Model file for the job. Use its own axes, mm. A direction names the side the tool comes from. Round coordinates to 2 decimals unless told otherwise and drop trailing zeros. Write each loop counter-clockwise with the first axis right and the second up, starting at its lowest first coordinate (ties: lowest second). Pieces come first, ordered by that corner, then holes. Notation, with made-up numbers: (24, 29.25) - (63, 29.25) arc R6 ccw to (63, 36.25) - close; hole circle Ø2 at (68.25, -39.75). An arc over 180 degrees is marked (long way). One line per item, written item: value.
from build123d import *

# Parameters (mm, degrees)
SKETCH1_W                       = 30
SKETCH1_H                       = 22
BOSS_EXTRUDE1_DEPTH             = 7
BOSS_EXTRUDE2_DEPTH             = 7
BOSS_EXTRUDE3_START             = 2
BOSS_EXTRUDE3_DEPTH             = 2
TAP_DRILL_FOR_M6X1_0_TAP2_D     = 5
TAP_DRILL_FOR_M6X1_0_TAP2_DEPTH = 8
TAP_DRILL_FOR_M6X1_0_TAP2_TIP   = 1.502151548


with BuildPart() as part:
    # Sketch1 → Boss-Extrude1 (new body)
    with BuildSketch(Plane(origin=(0, 0, 0), x_dir=(1, 0, 0), z_dir=(0, 1, 0))):
        with Locations((0, 3.5)):
            Rectangle(SKETCH1_W, SKETCH1_H)
        with BuildLine():
            ThreePointArc((-7.5, -2.5), (-10, -5), (-12.5, -2.5))
            Line((-12.5, -2.5), (-12.5, 2.5))
            ThreePointArc((-12.5, 2.5), (-10, 5), (-7.5, 2.5))
            Line((-7.5, 2.5), (-7.5, -2.5))
        make_face(mode=Mode.SUBTRACT)
        with BuildLine():
            ThreePointArc((12.5, -2.5), (10, -5), (7.5, -2.5))
            Line((7.5, -2.5), (7.5, 2.5))
            ThreePointArc((7.5, 2.5), (10, 5), (12.5, 2.5))
            Line((12.5, 2.5), (12.5, -2.5))
        make_face(mode=Mode.SUBTRACT)
    extrude(amount=BOSS_EXTRUDE1_DEPTH)

    # Sketch2 → Boss-Extrude2 (add)
    with BuildSketch(Plane(origin=(0, 0, -14.5), x_dir=(-1, 0, 0), z_dir=(0, 0, -1))):
        with BuildLine():
            Line((-15, 7), (15, 7))
            Line((15, 7), (43.5, 64))
            Line((43.5, 64), (43.5, 85))
            Line((43.5, 85), (27.855550733, 74.218014694))
            ThreePointArc((27.855550733, 74.218014694), (11.88121166, 46.405371431), (-19.795903133, 41.377147841))
            Line((-19.795903133, 41.377147841), (-30.5, 34))
            Line((-30.5, 34), (-15, 7))
        make_face()
    extrude(amount=-BOSS_EXTRUDE2_DEPTH)

    # Sketch3 → Boss-Extrude3 (add)
    with BuildSketch(Plane(origin=(0, 0, -14.5), x_dir=(-1, 0, 0), z_dir=(0, 0, -1)).offset(BOSS_EXTRUDE3_START)):
        with BuildLine():
            Line((-19.795903133, 41.377147841), (-30.5, 34))
            Line((-30.5, 34), (-25.504418015, 25.298018478))
            Line((-25.504418015, 25.298018478), (-3.837244639, 40.230800129))
            ThreePointArc((-3.837244639, 40.230800129), (-11.878974739, 39.935272554), (-19.795903133, 41.377147841))
        make_face()
        with BuildLine():
            Line((43.5, 85), (27.855550733, 74.218014694))
            ThreePointArc((27.855550733, 74.218014694), (26.38496828, 66.306368419), (23.246350456, 58.896521073))
            Line((23.246350456, 58.896521073), (43.5, 72.85511738))
            Line((43.5, 72.85511738), (43.5, 85))
        make_face()
    extrude(amount=-BOSS_EXTRUDE3_DEPTH)

    # Tap Drill for M6x1.0 Tap2
    with Locations(Plane(origin=(25.708369444, 37.302339978, 0), x_dir=(0.8233920666857286, -0.5674729108239484, 0), z_dir=(0.5674729108239484, 0.8233920666857286, 0))):
        with Locations((-75.680620934, 12), (-0.680620934, 12)):
            Hole(TAP_DRILL_FOR_M6X1_0_TAP2_D / 2, depth=TAP_DRILL_FOR_M6X1_0_TAP2_DEPTH)
            with Locations((0, 0, -(TAP_DRILL_FOR_M6X1_0_TAP2_DEPTH + TAP_DRILL_FOR_M6X1_0_TAP2_TIP / 2))):  # 118° drill point
                Cone(0, TAP_DRILL_FOR_M6X1_0_TAP2_D / 2, TAP_DRILL_FOR_M6X1_0_TAP2_TIP, mode=Mode.SUBTRACT)


solid = part.part
1. Mould opens along Z. For faces 1 (the face through (15, 3, -3)), 2 (the face through (0, 3, 7.5)), 3 (the face through (10, 3, 5)) say: released by +Z, released by -Z, zero draft, split by the parting line, or undercut.
Report:
face 1: zero draft
face 2: released by +Z
face 3: undercut
2. Band-saw the part on D-D on x = -10. Write the cut outline in (y, z).
Report:
outline: (0, -14.5) - (45.19, -14.5) - (45.19, -7.5) - (7, -7.5) - (7, -5) - (0, -5) - close; (0, 5) - (7, 5) - (7, 7.5) - (0, 7.5) - close
3. Tool access for faces 4 (the face through (-10, 3, -5)), 5 (the face through (-15, 3, -3)), 6 (the face through (0, 7, 0)): list every direction of +Z, -Z, +X, -X, +Y, -Y with a clear straight run to the whole face (end or side of a thin tool).
Report:
face 4: +Y, -Y
face 5: +Z, -Z, -X, -Y
face 6: +Z, +X, -X, +Y
4. Band-saw the part on B-B on z = -6.25. Write the cut outline in (x, y).
Report:
outline: (-15, 0) - (15, 0) - (15, 7) - (-15, 7) - close
5. Wall check: probe 1 along Z at (x, y) = (-31, 69.5); probe 2 along Z at (x, y) = (-17, 46); probe 3 along Y at (x, z) = (2, 1.25). Give the ranges that are in metal, low to high. Write a range as [from, to].
Report:
probe 1: [-16.5, -7.5]
probe 2: [-14.5, -7.5]
probe 3: [0, 7]
6. Drop flat-ended pins along their axis: pin 1 (8 mm diameter, centred on x = -24.5, y = 53.5, fed in from -Z); pin 2 (2 mm diameter, centred on x = -1, y = 11.5, fed in from +Z); pin 3 (6 mm diameter, centred on y = 20, z = -6.5, fed in from -X). Give the stop position or say it passes through.
Report:
pin 1: z = -14.5
pin 2: z = -7.5
pin 3: x = -22.91
7. Band-saw the part on A-A on x = 10. Write the cut outline in (y, z), plus the area to 3 significant figures.
Report:
outline: (0, -14.5) - (35.98, -14.5) - (35.98, -16.5) - (39.85, -16.5) - (39.85, -7.5) - (7, -7.5) - (7, -5) - (0, -5) - close; (0, 5) - (7, 5) - (7, 7.5) - (0, 7.5) - close
area: 322 mm²
8. Band-saw the part on C-C on y = 20.5. Write the cut outline in (x, z).
Report:
outline: (-21.75, -14.5) - (22.75, -14.5) - (22.75, -7.5) - (-21.75, -7.5) - close
